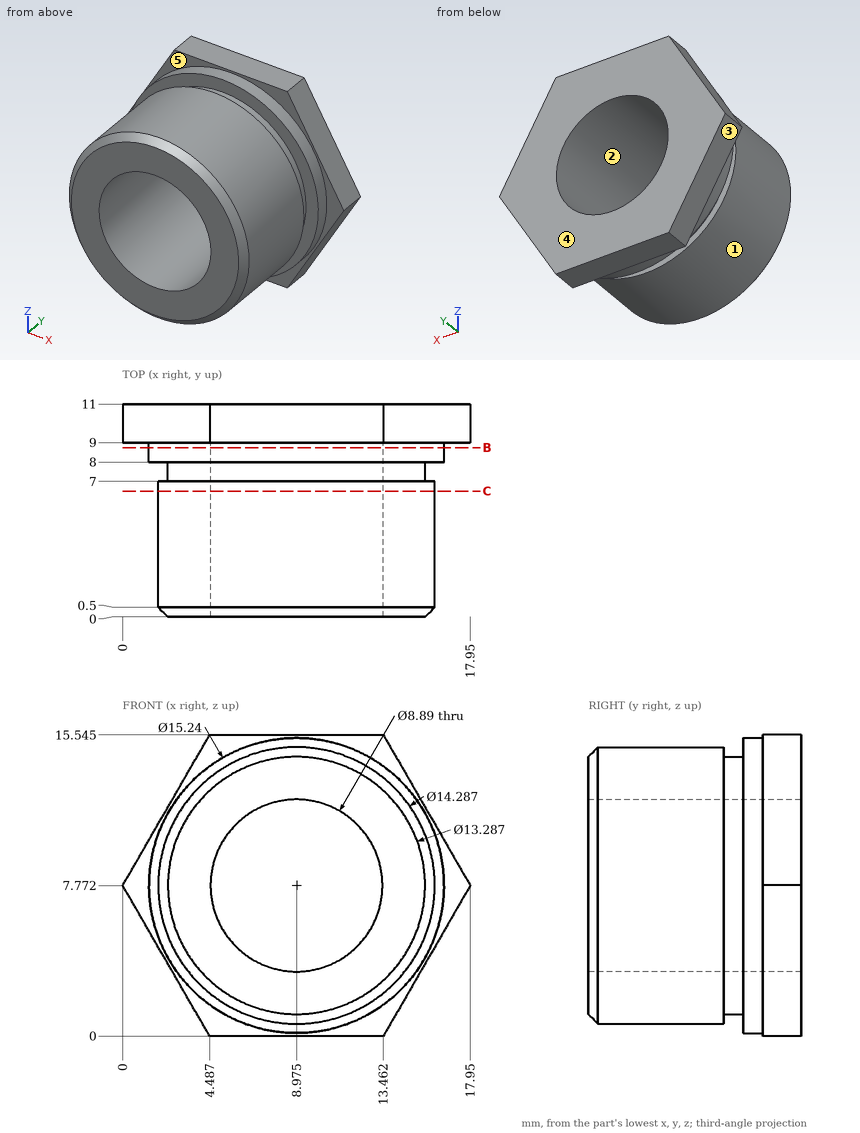
Verification items for this drawing (mm, ordinates from the low corner). A direction names the side the tool comes from. Give positions to 0.01 mm unless a question says otherwise; leave off trailing zeros. Loops run counter-clockwise (first coordinate to the right, second up) from the corner with the lowest first, then second, coordinate; pieces in that order, holes last. Notation, with made-up numbers: M 17.25,71.25 L 32.25,71.25 A23 cw 32.25,101.25 Z; hole C 14.25,12.25 d7. An arc over 180 degrees is marked long. Return JSON: item names as keys, results as strings. Group by question number.
1. Cross-section at C-C on y = 6.5. Record the boundary of the cut face in (x, z) (1 decimal).
2. Cross-section at B-B on y = 8.75. Record the boundary of the cut face in (x, z) (1 decimal), plus the area to 3 significant figures.
3. Go/stop test with a flat-tipped pin: pin 1 (5 mm diameter, centred on x = 12.5, y = 3, fed in from +Z). Record where the tip stops, or that it passes through.
4. Tool access check on the marked faces 4 and 5. Record the directions out of +Z, -Z, +X, -X, +Y, -Y that give a thin tool (end or side, any length) a straight path to the whole face; none if there is none.
5. Thickness scan on L1, parallel to X at y = 6.25, z = 5.5 (1 decimal); L2, parallel to Y at x = 6.25, z = 1.5 (1 decimal); L3, parallel to X at y = 9.75, z = 9.75 (1 decimal). Record the ranges inside material, lowest first.
6. Mould release check, pull along Z, two halves, no side actions. Record for the marked faces 1, 2 and 3: released by +Z, released by -Z, zero draft, split by the parting line, or undercut.
Return value:
{
 "1": {"outline": "C 9,7.8 d14.3; hole C 9,7.8 d8.9"},
 "2": {"outline": "C 9,7.8 d15.2; hole C 9,7.8 d8.9", "area": "120 mm^2"},
 "3": {"pin 1": "z = 14.84"},
 "4": {"face 4": "+Z, -Z, +X, -X, +Y", "face 5": "-Y"},
 "5": {"L1": "2.2 to 5.2, 12.8 to 15.7", "L2": "0.2 to 7, 8 to 11", "L3": "1.1 to 5, 13 to 16.8"},
 "6": {"face 1": "split by the parting line", "face 2": "undercut", "face 3": "released by -Z"}
}
